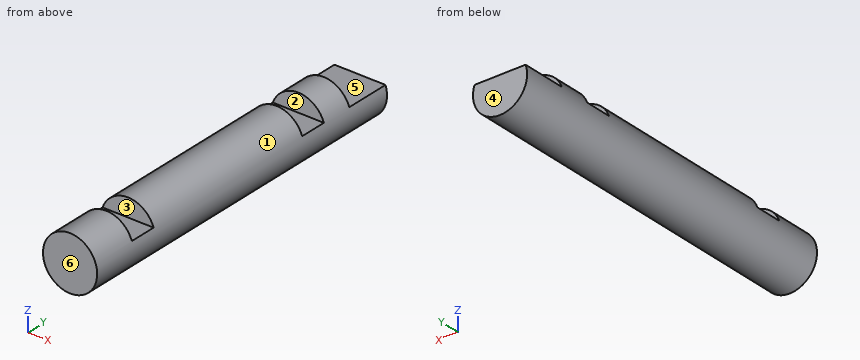
```python
from build123d import *

# Parameters (mm, degrees)
CROQUIS1_R                 = 3
SALIENTE_EXTRUIR1_DEPTH    = 20
CORTAR_EXTRUIR2_DEPTH      = 41.224370722
CORTAR_EXTRUIR2_DEPTH_BACK = 5
CROQUIS3_W                 = 8.224241852
CROQUIS3_H                 = 2
CROQUIS8_W                 = 6
CROQUIS8_H                 = 3
CORTAR_EXTRUIR4_DEPTH      = 10


with BuildPart() as part:
    # Croquis1 → Saliente-Extruir1 (new, symmetric)
    with BuildSketch(Plane(origin=(0, 0, 0), x_dir=(1, 0, 0), z_dir=(0, 1, 0))):
        with Locations(Location((0, 0, 0), (0, 0, 270))):
            Circle(CROQUIS1_R)
    extrude(amount=SALIENTE_EXTRUIR1_DEPTH, both=True)

    # Croquis3 → Cortar-Extruir2 (cut, two sides: drawn at the far end of the back side and taken through both)
    with BuildSketch(Plane(origin=(0, 20, 0), x_dir=(1, 0, 0), z_dir=(0, 1, 0)).offset(-CORTAR_EXTRUIR2_DEPTH_BACK)):
        with Locations((0.237694851, -2)):
            Rectangle(CROQUIS3_W, CROQUIS3_H)
    extrude(amount=CORTAR_EXTRUIR2_DEPTH + CORTAR_EXTRUIR2_DEPTH_BACK, mode=Mode.SUBTRACT)

    # Croquis8 → Cortar-Extruir4 (cut)
    with BuildSketch(Plane.XY.offset(1)):
        with Locations((0, 10)):
            Rectangle(CROQUIS8_W, CROQUIS8_H)
        with Locations((0, -13.5)):
            Rectangle(CROQUIS8_W, CROQUIS8_H)
    extrude(amount=CORTAR_EXTRUIR4_DEPTH, mode=Mode.SUBTRACT)


solid = part.part
```
Source: CAD feature listing. Evaluate the final solid. Frame: model axes, mm. Face numbers are marked on the shaded views. A direction names the side the tool comes from. Round coordinates to 2 decimals unless told otherwise and drop trailing zeros. Write each loop counter-clockwise with the first axis right and the second up, starting at its lowest first coordinate (ties: lowest second). Pieces come first, ordered by that corner, then holes. Notation, with made-up numbers: M -17,1 L 16,1 A18 ccw 16,5 Z; hole C 52,9 d5. An arc over 180 degrees is marked long. Answer as a JSON object with one key per item and string values. Group by question number.
(1) Mould query, pull axis Y, two halves, no side actions, for the marked faces 3, 4, 5 and 6. Classes: +Y half, -Y half, draft (parallel to the pull), parting line (faces both ways), or undercut.
(2) Section query C-C on y = -6. Output: boundary loops of the cut face in (x, z).
(3) Section query B-B on z = -1. Output: boundary loops of the cut face in (x, y), then the cut area to 3 significant figures.
(4) First-contact query: pin 1 (2 mm diameter, centred on x = 1.5, y = 13.5, fed in from +Z); pin 2 (0.9 mm diameter, centred on x = -1, y = 10, fed in from +Z); pin 3 (2 mm diameter, centred on x = -1, z = 2.5, fed in from +Y). Flat tips, straight axial feed; report the tip coordinate or a pass-through.
(5) Section query D-D on x = 1.65. Output: boundary loops of the cut face in (y, z).
(6) Reachability of the marked faces 1 and 2 from +Z, -Z, +X, -X, +Y, -Y: full face, straight path, thin tool, end or side. Return the list, or none.
(7) Section query A-A on x = 0. Output: boundary loops of the cut face in (y, z).
(8) Ray query, line 1 (X direction, y = -12.5, z = -0.1); line 2 (Z direction, x = -2.6, y = -14.5); line 3 (X direction, y = -3.5, z = -0.8). Return the intervals inside material, ascending. Write a range as [from, to].
Computed values:
{
 "1": {"face 3": "undercut", "face 4": "+Y half", "face 5": "draft", "face 6": "-Y half"},
 "2": {"outline": "C 0,0 d6"},
 "3": {"outline": "M -2.83,-20 L 2.83,-20 L 2.83,20 L -2.83,20 Z", "area": "226 mm^2"},
 "4": {"pin 1": "z = 2.96", "pin 2": "z = 1", "pin 3": "y = 15"},
 "5": {"outline": "M -20,-2.51 L 20,-2.51 L 20,1 L 15,1 L 15,2.51 L 11.5,2.51 L 11.5,1 L 8.5,1 L 8.5,2.51 L -12,2.51 L -12,1 L -15,1 L -15,2.51 L -20,2.51 Z"},
 "6": {"face 1": "+Y, -Y", "face 2": "+Z, +X, -X"},
 "7": {"outline": "M -20,-3 L 20,-3 L 20,1 L 15,1 L 15,3 L 11.5,3 L 11.5,1 L 8.5,1 L 8.5,3 L -12,3 L -12,1 L -15,1 L -15,3 L -20,3 Z"},
 "8": {"line 1": "[-3, 3]", "line 2": "[-1.5, 1]", "line 3": "[-2.89, 2.89]"}
}
